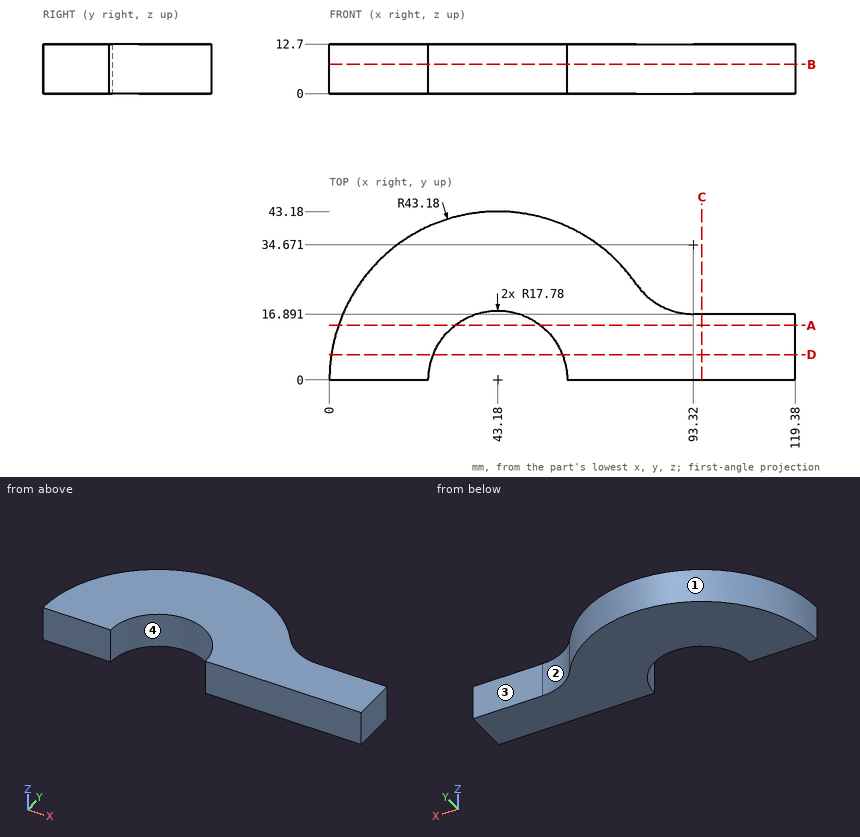
The drawing under review shows one solid part. Ordinate dimensions are in mm from its lowest x, y, z. Coordinates: 2 decimals unless noted, no trailing zeros. Order: outer loops, then holes, each group sorted by start corner. A loop starts at its lowest first (then second) coordinate and runs counter-clockwise, first axis right, second up. Notation, with made-up numbers: (44, -22) -> (77, -22) arc R8 cw to (77, -12) -> close; hole circle Ø6 at (74, -35). An arc over 180 degrees is marked (long way). Answer in a Markdown table with one row per item.
(1) Insertion check: pin 1 (6.5 mm diameter, centred on x = 113, z = 9, fed in from +Y); pin 2 (5 mm diameter, centred on y = 29.5, z = 8.5, fed in from -X); pin 3 (5 mm diameter, centred on y = 26, z = 6.5, fed in from -X) (1 decimal). Each pin has a flat end and moves straight along its axis. Give the tip position at first contact, or say it passes through.
Answers:
| item | result |
|---|---|
| pin 1 | y = 16.89 |
| pin 2 | x = 9.48 |
| pin 3 | x = 7 |
(2) Wall thickness on line 1 along X through (y, z) = (10, 3.75) (1 decimal); line 2 along X through (y, z) = (11.5, 8); line 3 along Y through (x, z) = (28, 4) (1 decimal): over which ranges is each line inside the solid? List them lowest first.
Answers:
| item | result |
|---|---|
| line 1 | 1.2 to 28.5, 57.9 to 119.4 |
| line 2 | 1.56 to 29.62, 56.74 to 119.38 |
| line 3 | 9.3 to 40.4 |
(3) Consider section B-B (z = 7.5). Write out the cut boundary in (x, y).
Answers:
| item | result |
|---|---|
| outline | (0, 0) -> (25.4, 0) arc R17.78 cw to (60.96, 0) -> (119.38, 0) -> (119.38, 16.89) -> (93.32, 16.89) arc R17.78 cw to (78.7, 24.56) arc R43.18 ccw to start |
(4) Consider section A-A (y = 14). Write out the cut boundary in (x, z).
Answers:
| item | result |
|---|---|
| outline | (2.33, 0) -> (32.22, 0) -> (32.22, 12.7) -> (2.33, 12.7) -> close; (54.14, 0) -> (119.38, 0) -> (119.38, 12.7) -> (54.14, 12.7) -> close |
(5) Consider section C-C (x = 95.5). Write out the cut boundary in (y, z).
Answers:
| item | result |
|---|---|
| outline | (0, 0) -> (16.89, 0) -> (16.89, 12.7) -> (0, 12.7) -> close |
(6) The part is to be moulded in two halves that separate along X. For the marked faces 1, 2, 3 and 4, say which applies: +X half, -X half, draft (parallel to the pull), parting line (faces both ways), or undercut.
Answers:
| item | result |
|---|---|
| face 1 | parting line |
| face 2 | +X half |
| face 3 | draft |
| face 4 | undercut |
(7) Consider section D-D (y = 6.5). Write out the cut boundary in (x, z).
Answers:
| item | result |
|---|---|
| outline | (0.49, 0) -> (26.63, 0) -> (26.63, 12.7) -> (0.49, 12.7) -> close; (59.73, 0) -> (119.38, 0) -> (119.38, 12.7) -> (59.73, 12.7) -> close |
